Print and shaded views of the part. All mm, measured from the part's lowest x, y and z. A direction names the side the tool comes from. Round coordinates to 2 decimals unless told otherwise and drop trailing zeros. Write each loop counter-clockwise with the first axis right and the second up, starting at its lowest first coordinate (ties: lowest second). Pieces come first, ordered by that corner, then holes.
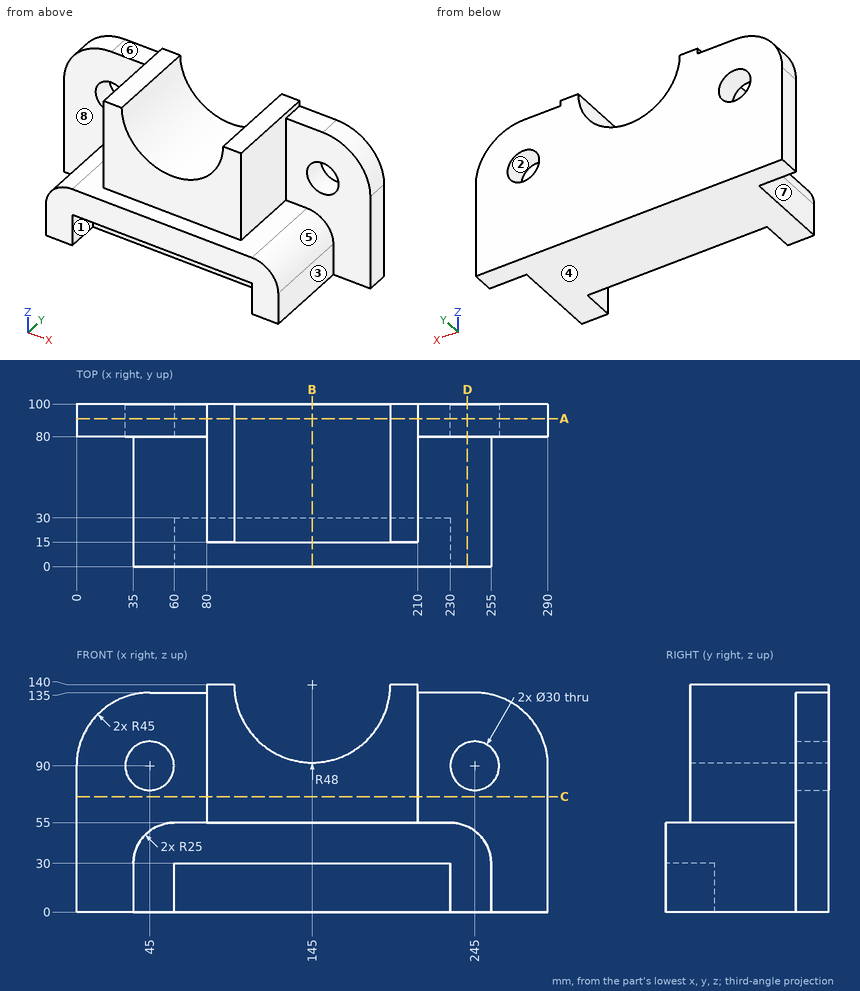
1) Slice it at D-D (x = 240.5). Write the cut outline in (y, z), plus the area to 3 significant figures.
Results:
outline: (0, 0) - (100, 0) - (100, 75.69) - (80, 75.69) - (80, 52.69) - (0, 52.69) - close; (80, 104.31) - (100, 104.31) - (100, 135) - (80, 135) - close
area: 6,340 mm2
2) Slice it at A-A (y = 91). Write the cut outline in (x, z), plus the area to 3 significant figures.
Results:
outline: (0, 0) - (290, 0) - (290, 90) arc R45 ccw to (245, 135) - (210, 135) - (210, 140) - (193, 140) arc R48 cw to (97, 140) - (80, 140) - (80, 135) - (45, 135) arc R45 ccw to (0, 90) - close; hole circle Ø30 at (45, 90); hole circle Ø30 at (245, 90)
area: 33,900 mm2
3) Wall check: L1, parallel to Z at x = 45, y = 87; L2, parallel to Y at x = 70.5, z = 92; L3, parallel to Y at x = 148, z = 20.5. Give the ranges that are in metal, low to high.
Results:
L1: z = 0 to 75, 105 to 135
L2: y = 80 to 100
L3: y = 30 to 100
4) Mould opens along X. For the marked faces 1, 2, 3 and 4 say: released by +X, released by -X, zero draft, split by the parting line, or undercut.
Results:
face 1: undercut
face 2: undercut
face 3: released by +X
face 4: zero draft
5) Slice it at C-C (z = 71). Write the cut outline in (x, y).
Results:
outline: (0, 80) - (80, 80) - (80, 15) - (210, 15) - (210, 80) - (290, 80) - (290, 100) - (0, 100) - close
6) Slice it at B-B (x = 145). Write the cut outline in (y, z).
Results:
outline: (0, 30) - (30, 30) - (30, 0) - (100, 0) - (100, 92) - (15, 92) - (15, 55) - (0, 55) - close
7) Which spindle directions (+Z, -Z, +X, -X, +Y, -Y) get a long thin tool onto all of the face, cutting with end or side? Do the marked faces 5, 6, 7 and 8. Say none if no direction does.
Results:
face 5: +Z, +X, -Y
face 6: +Z, -X, +Y, -Y
face 7: +Z, -Z, -X, -Y
face 8: +Z, -X, -Y
8) Pin check, flat tips, straight feed: pin 1 Ø24 at (y, z) = (54.5, 18.5) entering from +X; pin 2 Ø24 at (y, z) = (38, 21) entering from -X; pin 3 Ø1 at (x, y) = (152, 25) entering from +Z; pin 4 Ø1 at (x, y) = (158, 40.5) entering from -Z. Stop position of each tip, or through.
Results:
pin 1: stops at x = 255
pin 2: stops at x = 35
pin 3: stops at z = 92.59
pin 4: stops at z = 0
